Can you work these out from the model? Positions are in its coordinate system, mm. A direction names the side the tool comes from. Give positions to 0.01 mm unless a question says otherwise; leave off trailing zeros. Loops run counter-clockwise (first coordinate to the right, second up) from the corner with the lowest first, then second, coordinate; pieces in that order, holes last. Notation, with made-up numbers: M -34,42.25 L 10,42.25 A19 ccw 10,46.25 Z; hole C -16,2.25 d7. An arc over 180 degrees is marked long. Answer as a JSON object with one key per item and string values.
```python
from build123d import *

# Parameters (mm, degrees)
SKETCH2_W                    = 254
SKETCH2_H                    = 254
SKETCH2_R                    = 3.175
BASE_FLANGE1_DEPTH           = 6.35
EDGE_FLANGE1_STRIP_W         = 38.1
EDGE_FLANGE1_STRIP_H         = 6.35
EDGE_FLANGE1_STRIP_CUT_DEPTH = 254
EDGE_FLANGE1_DEPTH           = 254
SKETCH10_R                   = 57.15
CUT_EXTRUDE1_DEPTH           = 437.305538012
SKETCH12_R                   = 3.175
CUT_EXTRUDE2_DEPTH           = 433.639624861


# Sheet-metal steps are written as plain solids
with BuildPart() as part:
    # Sketch2 → Base-Flange1 (new body)
    with BuildSketch(Plane(origin=(0, 0, 0), x_dir=(1, 0, 0), z_dir=(0, 1, 0))):
        with Locations((127, 127)):
            Rectangle(SKETCH2_W, SKETCH2_H)
        with Locations(Location((190.5, 152.4, 0), (0, 0, 270))):
            Circle(SKETCH2_R, mode=Mode.SUBTRACT)
        with Locations(Location((127, 152.4, 0), (0, 0, 270))):
            Circle(SKETCH2_R, mode=Mode.SUBTRACT)
        with Locations(Location((63.5, 152.4, 0), (0, 0, 270))):
            Circle(SKETCH2_R, mode=Mode.SUBTRACT)
        with Locations(Location((127, 101.6, 0), (0, 0, 270))):
            Circle(SKETCH2_R, mode=Mode.SUBTRACT)
        with Locations(Location((63.5, 101.6, 0), (0, 0, 270))):
            Circle(SKETCH2_R, mode=Mode.SUBTRACT)
        with Locations(Location((190.5, 101.6, 0), (0, 0, 270))):
            Circle(SKETCH2_R, mode=Mode.SUBTRACT)
    extrude(amount=-BASE_FLANGE1_DEPTH)

    # Edge-Flange1 strip (across the edge) → Edge-Flange1 strip cut (cut)
    with BuildSketch(Plane.XY.offset(-254)):
        with Locations((-6.35, -3.175)):
            Rectangle(EDGE_FLANGE1_STRIP_W, EDGE_FLANGE1_STRIP_H)
    extrude(amount=EDGE_FLANGE1_STRIP_CUT_DEPTH, mode=Mode.SUBTRACT)

    # Edge-Flange1 section (across the edge) → Edge-Flange1 (add)
    with BuildSketch(Plane.XY.offset(-254)):
        with BuildLine():
            Line((0, 6.35), (0, 247.65))
            Line((0, 247.65), (6.35, 247.65))
            Line((6.35, 247.65), (6.35, 6.35))
            ThreePointArc((6.35, 6.35), (8.209871939, 1.859871939), (12.7, 0))
            Line((12.7, 0), (12.7, -6.35))
            ThreePointArc((12.7, -6.35), (3.719743879, -2.630256121), (0, 6.35))
        make_face()
    extrude(amount=EDGE_FLANGE1_DEPTH)

    # Sketch10 → Cut-Extrude1 (cut, through all)
    with BuildSketch(Plane.ZY):
        with Locations(Location((-127, 120.65, 0), (0, 0, 270))):
            Circle(SKETCH10_R)
    extrude(amount=-CUT_EXTRUDE1_DEPTH, mode=Mode.SUBTRACT)

    # Sketch12 → Cut-Extrude2 (cut, through all)
    with BuildSketch(Plane(origin=(6.35, 0, 0), x_dir=(0, 0, -1), z_dir=(1, 0, 0))):
        with Locations(Location((75.296364232, 57.803324087, 0), (0, 0, 90))):
            Circle(SKETCH12_R)
        with Locations(Location((46.721364232, 107.296675913, 0), (0, 0, 90))):
            Circle(SKETCH12_R)
        with Locations(Location((98.425, 196.85, 0), (0, 0, 90))):
            Circle(SKETCH12_R)
        with Locations(Location((155.575, 196.85, 0), (0, 0, 90))):
            Circle(SKETCH12_R)
        with Locations(Location((178.703635768, 57.803324087, 0), (0, 0, 90))):
            Circle(SKETCH12_R)
        with Locations(Location((207.278635768, 107.296675913, 0), (0, 0, 90))):
            Circle(SKETCH12_R)
    extrude(amount=-CUT_EXTRUDE2_DEPTH, mode=Mode.SUBTRACT)


solid = part.part
```
1) Will these pins go through, and if not, where does the flat tip stop? pin 1 Ø10 at (y, z) = (107.3, -207.28) entering from -X; pin 2 Ø7.5 at (x, z) = (190.5, -101.6) entering from +Y; pin 3 Ø10 at (y, z) = (82.5, -76.5) entering from +X.
Answer list:
{"pin 1": "x = 0", "pin 2": "y = 0", "pin 3": "x = 6.35"}
2) Suppose I cut it at C-C, the plane z = -32.5. Write out the boundary of the cut face in (x, y).
Answer list:
{"outline": "M 0,6.35 A12.7 ccw 12.7,-6.35 L 254,-6.35 L 254,0 L 12.7,0 A6.35 cw 6.35,6.35 L 6.35,247.65 L 0,247.65 Z"}
3) If we mould it in two halves opening along Z, with no side actions, what happens to faces 1 (the cylindrical face through (3.13, 67.86, -148.89)), 2 (the flat face through (0, 179, -129)), 3 (the flat face through (5, 65, 0))? For each: +Z half, -Z half, draft (parallel to the pull), parting line (faces both ways), or undercut.
Answer list:
{"face 1": "undercut", "face 2": "draft", "face 3": "+Z half"}
4) Suppose I cut it at D-D, the plane x = 52.5. Write out the boundary of the cut face in (y, z).
Answer list:
{"outline": "M -6.35,-254 L 0,-254 L 0,0 L -6.35,0 Z"}
5) Suppose I cut it at B-B, the plane y = 120.65. Write out the boundary of the cut face in (x, z), and give its area (3 significant figures).
Answer list:
{"outline": "M 0,-254 L 6.35,-254 L 6.35,-184.15 L 0,-184.15 Z; M 0,-69.85 L 6.35,-69.85 L 6.35,0 L 0,0 Z", "area": "887 mm^2"}
6) For faces 4 (the flat face through (5, 65, -254)), 5 (the flat face through (132, 0, -129)), which set-ups out of +Z, -Z, +X, -X, +Y, -Y let a thin tool reach every point of the face, with its end or its side?
Answer list:
{"face 4": "-Z, +X, -X, +Y, -Y", "face 5": "+Z, -Z, +X, +Y"}
7) Please list where these lines run through material, in increasing order: line 1 along Z through (x, y) = (4, 196.85); line 2 along Z through (x, y) = (190, -3); line 3 along X through (y, z) = (-2, -152.4) (3 decimals). Write a range as from..to.
Answer list:
{"line 1": "-254..-158.75, -152.4..-101.6, -95.25..0", "line 2": "-254..-155.54, -149.26..-104.74, -98.46..0", "line 3": "3.131..60.325, 66.675..123.825, 130.175..187.325, 193.675..254"}
8) Suppose I cut it at A-A, the plane z = -127. Write out the boundary of the cut face in (x, y).
Answer list:
{"outline": "M 0,6.35 A12.7 ccw 12.7,-6.35 L 254,-6.35 L 254,0 L 12.7,0 A6.35 cw 6.35,6.35 L 6.35,63.5 L 0,63.5 Z; M 0,177.8 L 6.35,177.8 L 6.35,247.65 L 0,247.65 Z"}
